Source: CAD feature listing. Evaluate the final solid. Frame: model axes, mm. Face numbers are marked on the shaded views. A direction names the side the tool comes from. Give positions to 0.01 mm unless a question says otherwise; leave off trailing zeros. Loops run counter-clockwise (first coordinate to the right, second up) from the corner with the lowest first, then second, coordinate; pieces in that order, holes last. Notation, with made-up numbers: (80, 18) -> (112, 18) arc R17 ccw to (112, 51) -> close; hole circle Ø1 at (7.25, -20). An arc over 180 degrees is marked (long way). Return JSON: item names as keys, results as strings. Group by question number.
(1) Cut plane A-A on z = 6.15. Return loops of the section in (x, y).
(2) Cut plane D-D on x = 18. Return loops of the section in (y, z).
(3) Pin query (flat end, axial travel): pin 1 (4 mm diameter, centred on y = 21.5, z = 5, fed in from -X); pin 2 (5 mm diameter, centred on x = 18, z = 6.15, fed in from +Y). Return the tip coordinate at first contact, or that it passes through.
(4) Draft query along Y for the marked faces 1, 2 and 3. Return one class per face: released by +Y, released by -Y, zero draft, split by the parting line, or undercut.
(5) Cut plane B-B on y = 5.5. Return loops of the section in (x, z).
(6) Access query for the marked faces 4 and 5. Directions: +Z, -Z, +X, -X, +Y, -Y. A direction counts if a zero-diameter tool reaches every point of the face in a straight line with its end or side. Return the directions, or none.
(7) Cut plane C-C on x = 23. Return loops of the section in (y, z).
(8) Ray query, line 1 (Y direction, x = 27.42, z = 7.75); line 2 (Z direction, x = 18, y = 30); line 3 (Y direction, x = 12.5, z = 10.75). Return the intervals inside material, ascending. Write a range as from..to.
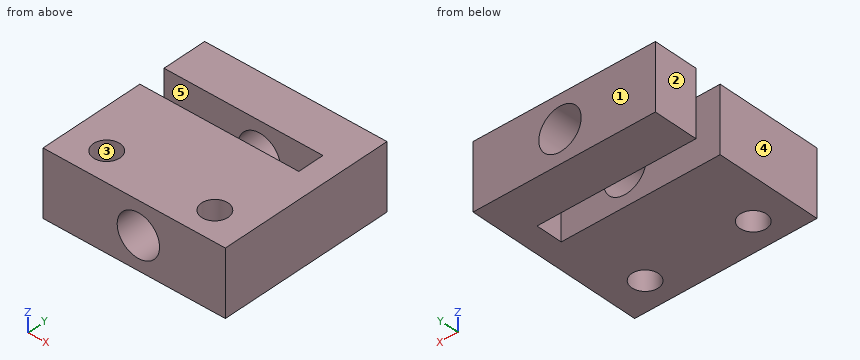
```python
from build123d import *

# Parameters (mm, degrees)
SKETCH1_R           = 2.5
BOSS_EXTRUDE1_DEPTH = 12.3
SKETCH2_R           = 4
CUT_EXTRUDE1_DEPTH  = 34.42


with BuildPart() as part:
    # Sketch1 → Boss-Extrude1 (new body)
    with BuildSketch(Plane.XY):
        Polygon((0, 25.02), (30, 25.02), (30, 20.02), (0, 20.02), (0, 0), (34.42, 0), (34.42, 33.42), (0, 33.42), align=None)
        with Locations((27.42, 5.5)):
            Circle(SKETCH1_R, mode=Mode.SUBTRACT)
        with Locations((7, 5.5)):
            Circle(SKETCH1_R, mode=Mode.SUBTRACT)
    extrude(amount=BOSS_EXTRUDE1_DEPTH)

    # Sketch2 → Cut-Extrude1 (cut, through all)
    with BuildSketch(Plane(origin=(0, 0, 0), x_dir=(-1, 0, 0), z_dir=(0, -1, 0))):
        with Locations((-18, -6.15)):
            Circle(SKETCH2_R)
    extrude(amount=-CUT_EXTRUDE1_DEPTH, mode=Mode.SUBTRACT)


solid = part.part
```
Answers:
{
 "1": {"outline": "(0, 0) -> (14, 0) -> (14, 20.02) -> (0, 20.02) -> close; (0, 25.02) -> (14, 25.02) -> (14, 33.42) -> (0, 33.42) -> close; (22, 0) -> (34.42, 0) -> (34.42, 33.42) -> (22, 33.42) -> (22, 25.02) -> (30, 25.02) -> (30, 20.02) -> (22, 20.02) -> close; hole circle Ø5 at (7, 5.5); hole circle Ø5 at (27.42, 5.5)"},
 "2": {"outline": "(0, 0) -> (20.02, 0) -> (20.02, 2.15) -> (0, 2.15) -> close; (0, 10.15) -> (20.02, 10.15) -> (20.02, 12.3) -> (0, 12.3) -> close; (25.02, 0) -> (33.42, 0) -> (33.42, 2.15) -> (25.02, 2.15) -> close; (25.02, 10.15) -> (33.42, 10.15) -> (33.42, 12.3) -> (25.02, 12.3) -> close"},
 "3": {"pin 1": "x = 0", "pin 2": "through"},
 "4": {"face 1": "released by +Y", "face 2": "zero draft", "face 3": "undercut"},
 "5": {"outline": "(0, 0) -> (4.5, 0) -> (4.5, 12.3) -> (0, 12.3) -> close; (9.5, 0) -> (24.92, 0) -> (24.92, 12.3) -> (9.5, 12.3) -> close; (29.92, 0) -> (34.42, 0) -> (34.42, 12.3) -> (29.92, 12.3) -> close; hole circle Ø8 at (18, 6.15)"},
 "6": {"face 4": "+Z, -Z, -X, +Y, -Y", "face 5": "+Z, -Z, -X"},
 "7": {"outline": "(0, 0) -> (20.02, 0) -> (20.02, 12.3) -> (0, 12.3) -> close; (25.02, 0) -> (33.42, 0) -> (33.42, 12.3) -> (25.02, 12.3) -> close"},
 "8": {"line 1": "0..3, 8..20.02, 25.02..33.42", "line 2": "0..2.15, 10.15..12.3", "line 3": "0..20.02, 25.02..33.42"}
}
